from build123d import *

# Parameters (mm, degrees)
SKETCH_W     = 34.6
SKETCH_H     = 58.8
PAD_DEPTH    = 4
PAD001_DEPTH = 17.6
PAD003_DEPTH = 59.8
PAD004_DEPTH = 3.5
POCKET_DEPTH = 10


with BuildPart() as part:
    # Sketch → Pad (new body)
    with BuildSketch(Plane.XY.offset(-2)):
        Rectangle(SKETCH_W, SKETCH_H)
    extrude(amount=PAD_DEPTH)

    # Sketch001 → Pad001 (join)
    with BuildSketch(Plane.XY.offset(2)):
        Polygon((-15.3, -29.4), (-15.3, 27.4), (15.3, 27.4), (15.3, -29.4), (17.3, -29.4), (17.3, 29.4), (-17.3, 29.4), (-17.3, -29.4), align=None)
    extrude(amount=PAD001_DEPTH)

    # Sketch003 → Pad003 (join)
    with BuildSketch(Plane.XZ.offset(30.4)):
        Polygon((-15.3625, 20.45), (-16.1125, 20.45), (-16.1125, 0.1), (16.1125, 0.1), (16.1125, 20.45), (15.3625, 20.45), (15.3625, 1.9), (-15.3625, 1.9), align=None)
    extrude(amount=-PAD003_DEPTH)

    # Sketch004 → Pad004 (join)
    with BuildSketch(Plane.XZ.offset(-27.4)):
        Polygon((-15.3, 19.6), (-15.3, 16.3), (-10, 19.6), align=None)
        Polygon((15.3, 19.6), (15.3, 16.3), (10, 19.6), align=None)
    extrude(amount=PAD004_DEPTH)

    # Sketch005 → Pocket (cut, symmetric)
    with BuildSketch(Plane.YZ):
        Polygon((20, 0), (20, -2), (10, -2), align=None)
    extrude(amount=POCKET_DEPTH, both=True, mode=Mode.SUBTRACT)


solid = part.part
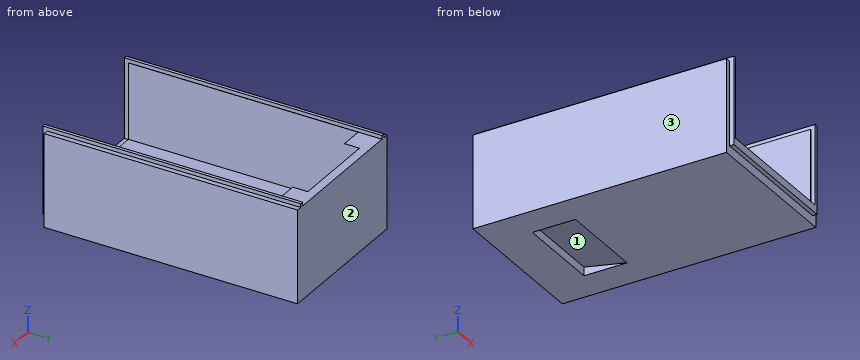
Source: CAD feature listing. Evaluate the final solid. Frame: model axes, mm. Face numbers are marked on the shaded views. Round coordinates to 2 decimals unless told otherwise and drop trailing zeros. Order: outer loops, then holes, each group sorted by start corner. A loop starts at its lowest first (then second) coordinate and runs counter-clockwise, first axis right, second up. Notation, with made-up numbers: (65, 43.5) - (76, 43.5) arc R20 ccw to (76, 61.5) - close; hole circle Ø2 at (89, 5). An arc over 180 degrees is marked (long way). Use a Markdown table: item, result. Add a question column.
1. Section query B-B (y = 22.5). Return the cut outline in (x, z), then the cut area to 3 significant figures.
2. Section query C-C (x = -3.5). Return the cut outline in (y, z), then the cut area to 3 significant figures.
3. Section query A-A (z = 15). Return the cut outline in (x, y).
4. First-contact query: pin 1 (4 mm diameter, centred on x = 9, y = -8.5, fed in from +Z); pin 2 (4 mm diameter, centred on x = 5, z = 16.5, fed in from -Y); pin 3 (1 mm diameter, centred on x = -13.5, z = 18.5, fed in from -Y). Flat tips, straight axial feed; report the tip coordinate or a pass-through.
5. Mould query, pull axis X, two halves, no side actions, for the marked faces 1, 2 and 3. Classes: +X half, -X half, draft (parallel to the pull), parting line (faces both ways), or undercut.
6. Line query: probe 1 along X at (y, z) = (-22.5, 4.25); probe 2 along Y at (x, z) = (-15, 6.5); probe 3 along Z at (x, y) = (4, 4.5). Output: solid intervals per line, ascending.
Derived:
| question | item | result |
|---|---|---|
| 1 | outline | (-17.3, -2) - (17.3, -2) - (17.3, 19.6) - (16.11, 19.6) - (16.11, 20.45) - (15.36, 20.45) - (15.36, 19.6) - (15.3, 19.6) - (15.3, 2) - (-15.3, 2) - (-15.3, 19.6) - (-15.36, 19.6) - (-15.36, 20.45) - (-16.11, 20.45) - (-16.11, 19.6) - (-17.3, 19.6) - close |
| 1 | area | 210 mm2 |
| 2 | outline | (-30.4, 0.1) - (-29.4, 0.1) - (-29.4, -2) - (10, -2) - (20, 0) - (20, -2) - (29.4, -2) - (29.4, 19.6) - (27.4, 19.6) - (27.4, 2) - (-29.4, 2) - (-29.4, 1.9) - (-30.4, 1.9) - close |
| 2 | area | 262 mm2 |
| 3 | outline | (-17.3, -29.4) - (-16.11, -29.4) - (-16.11, -30.4) - (-15.36, -30.4) - (-15.36, -29.4) - (-15.3, -29.4) - (-15.3, 27.4) - (15.3, 27.4) - (15.3, -29.4) - (15.36, -29.4) - (15.36, -30.4) - (16.11, -30.4) - (16.11, -29.4) - (17.3, -29.4) - (17.3, 29.4) - (-17.3, 29.4) - close |
| 4 | pin 1 | z = 2 |
| 4 | pin 2 | y = 27.4 |
| 4 | pin 3 | y = 23.9 |
| 5 | face 1 | undercut |
| 5 | face 2 | draft |
| 5 | face 3 | -X half |
| 6 | probe 1 | -17.3 to -15.3, 15.3 to 17.3 |
| 6 | probe 2 | 27.4 to 29.4 |
| 6 | probe 3 | -2 to 2 |
